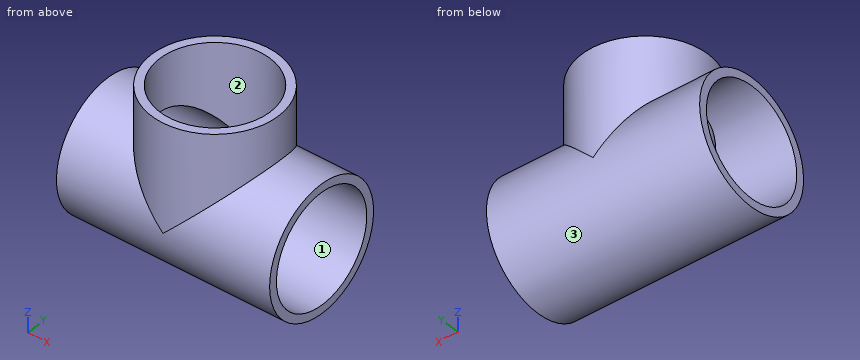
Autodesk Inventor part; units mm, degrees
ref_plane "YZ Plane" through (0, 0, 0) normal (1, 0, 0) x (0, 1, 0)
ref_plane "XZ Plane" through (0, 0, 0) normal (0, 1, 0) x (-1, 0, 0)
ref_plane "XY Plane" through (0, 0, 0) normal (0, 0, 1) x (1, 0, 0)
sketch "Sketch1" plane through (0, 0, 0) normal (1, 0, 0) x (0, 1, 0)
  circle A0 centre (0, 0) radius 84.15
  dimension "d0" = 168.3
extrude "Extrude1" add sketch "Sketch1" along normal blind 286
sketch "Sketch2" plane through (0, 0, 0) normal (0, 0, 1) x (1, 0, 0)
  line L0 (0, 84.15) -> (0, -84.15)
  line L1 (286, 84.15) -> (286, -84.15)
  line L2 (0, 0) -> (286, 0) construction
  circle A0 centre (143, 0) radius 84.15
  dimension "d3" = 168.3
extrude "Extrude2" add sketch "Sketch2" along normal blind 143
sketch "Sketch3" plane through (0, 0, 0) normal (-1, 0, 0) x (0, 0, 1)
  circle A0 centre (0, 0) radius 84.15
  circle A1 centre (0, 0) radius 73.15
  dimension "d6" = 146.3
extrude "Extrude3" cut sketch "Sketch3" against normal through all contours A1
sketch "Sketch4" plane through (143, 0, 143) normal (0, 0, 1) x (1, 0, 0)
  circle A0 centre (0, 0) radius 84.15
  circle A1 centre (0, 0) radius 73.15
  dimension "d9" = 146.3
extrude "Extrude4" cut sketch "Sketch4" against normal up to next contours A1
equation "\"d0\" = d"
equation "\"d1\" = 2 * a"
equation "\"d3\" = d"
equation "\"d4\" = a"
equation "\"d6\" = d - 2 * s1"
equation "\"d7\" = a"
equation "\"d9\" = d - 2 * s1"
equation "\"d10\" = a"
equation "\"d\" = 168.3"
equation "\"s1\" = 11"
equation "\"a\" = 143"
equation "\"Size_Designation\" = 1.2345"
properties part number "DIN 2615-1 Tee 168.3 x 11 S" material "Steel"
Check sheet for the modelled part. Datum: model origin and axes. Units: mm. Face numbers are marked on the shaded views. Coordinates: 2 decimals unless noted, no trailing zeros. Write each loop counter-clockwise with the first axis right and the second up, starting at its lowest first coordinate (ties: lowest second). Pieces come first, ordered by that corner, then holes.
Item 1: Cross-section at B-B on x = 143. Record the boundary of the cut face in (y, z), then the cut area to 3 significant figures.
Numbers:
outline: (-84.15, 0) arc R84.15 ccw to (84.15, 0) - (84.15, 143) - (73.15, 143) - (73.15, 0) arc R73.15 cw to (-73.15, 0) - (-73.15, 143) - (-84.15, 143) - close
area: 5,860 mm2
Item 2: Depth check by flat-ended pin: pin 1 Ø1 at (x, z) = (49, -54.5) entering from -Y; pin 2 Ø5 at (x, z) = (58, 73.5) entering from -Y; pin 3 Ø10 at (x, z) = (83.5, -61) entering from -Y. Enter the tip coordinate at first touch or a pass-through.
Numbers:
pin 1: stops at y = -64.54
pin 2: stops at y = -45.17
pin 3: stops at y = -62.81
Item 3: Cross-section at C-C on z = -43. Record the boundary of the cut face in (x, y).
Numbers:
outline: (0, -72.33) - (286, -72.33) - (286, -59.18) - (0, -59.18) - close; (0, 59.18) - (286, 59.18) - (286, 72.33) - (0, 72.33) - close
Item 4: Cross-section at D-D on x = 28. Record the boundary of the cut face in (y, z).
Numbers:
outline: circle Ø168.3 at (0, 0); hole circle Ø146.3 at (0, 0)
Item 5: Scan lines: probe 1 along Y at (x, z) = (143, 95); probe 2 along Z at (x, y) = (36, -2); probe 3 along X at (y, z) = (0, 94). Record each from-to range of solid material in increasing order.
Numbers:
probe 1: y = -84.15 to -73.15, 73.15 to 84.15
probe 2: z = -84.13 to -73.12, 73.12 to 84.13
probe 3: x = 58.85 to 69.85, 216.15 to 227.15
Item 6: Cross-section at A-A on y = 0. Record the boundary of the cut face in (x, z).
Numbers:
outline: (0, -84.15) - (286, -84.15) - (286, -73.15) - (0, -73.15) - close; (0, 73.15) - (69.85, 73.15) - (69.85, 143) - (58.85, 143) - (58.85, 84.15) - (0, 84.15) - close; (216.15, 73.15) - (286, 73.15) - (286, 84.15) - (227.15, 84.15) - (227.15, 143) - (216.15, 143) - close
Item 7: Mould release check, pull along Y, two halves, no side actions. Record for the marked faces 1, 2 and 3: released by +Y, released by -Y, zero draft, split by the parting line, or undercut.
Numbers:
face 1: undercut
face 2: undercut
face 3: split by the parting line
